Autodesk Fusion 360 part; units mm, degrees
sketch "Sketch1" plane through (0, 0, 0) normal (0, 0, 1) x (1, 0, 0)
  line L0 (0, 0) -> (70, 0)
  line L1 (70, 0) -> (70, 70)
  line L2 (70, 70) -> (0, 70)
  line L3 (0, 70) -> (0, 0)
  circle A0 centre (7.5, 62.5) radius 1.75
  circle A1 centre (62.5, 62.5) radius 1.75
  circle A2 centre (7.5, 7.5) radius 1.75
  circle A3 centre (62.5, 7.5) radius 1.75
  dimension "d1" = 70
  dimension "d2" = 70
  dimension "d3" = 3.5
  dimension "d4" = 7.5
  dimension "d5" = 7.5
  dimension "d8" = 55
  dimension "d9" = -55
extrude "Extrude1" add sketch "Sketch1" along normal blind 5
sketch "Sketch2" plane through (0, 0, 5) normal (0, 0, 1) x (-1, 0, 0)
  circle A0 centre (-62.5, -7.5) radius 1.75
  circle A1 centre (-7.5, -62.5) radius 1.75
  circle A2 centre (-7.5, -7.5) radius 1.75
  circle A3 centre (-62.5, -62.5) radius 1.75
  line L0 (0, -70) -> (0, 0)
  line L1 (0, 0) -> (-70, 0)
  line L2 (-70, 0) -> (-70, -70)
  line L3 (-70, -70) -> (0, -70)
  circle A4 centre (-35, -35) radius 11.4
  dimension "d12" = 22.8
extrude "Extrude2" cut sketch "Sketch2" against normal blind 5 contours A4
sketch "Sketch3" plane through (0, 0, 5) normal (0, 0, 1) x (-1, 0, 0)
  circle A0 centre (-35, -35) radius 11.4
  circle A1 centre (-62.5, -7.5) radius 1.75
  circle A2 centre (-7.5, -62.5) radius 1.75
  circle A3 centre (-7.5, -7.5) radius 1.75
  circle A4 centre (-62.5, -62.5) radius 1.75
  line L0 (0, -70) -> (0, 0)
  line L1 (0, 0) -> (-70, 0)
  line L2 (-70, 0) -> (-70, -70)
  line L3 (-70, -70) -> (0, -70)
  circle A5 centre (-35, -35) radius 16
  dimension "d15" = 32
extrude "Extrude3" add sketch "Sketch3" along normal blind 15 contours A0 | A5
sketch "Sketch4" plane through (0, 0, 20) normal (0, 0, 1) x (-1, 0, 0)
  circle A0 centre (-35, -35) radius 16
  circle A1 centre (-35, -35) radius 4.5
  dimension "d18" = 9
extrude "Extrude4" cut sketch "Sketch4" against normal blind 45 contours A1
sketch "Sketch5" plane through (0, 0, 20) normal (0, 0, 1) x (-1, 0, 0)
  circle A0 centre (-35, -35) radius 4.5
  circle A1 centre (-35, -35) radius 16
  circle A2 centre (-35, -35) radius 11.4
  dimension "d21" = 22.8
extrude "Extrude5" cut sketch "Sketch5" against normal blind 6 contours A2
extrude "Extrude6" add 1 faces at (25.9592, 35.7899, 5) along direction (0, 0, -1) blind 3.5
chamfer "Chamfer1" distance 6 angle 45 2 edges at (39.1955, 36.6273, 14) (39.1955, 36.6273, 1.5)
fillet "Fillet2" radius 65 1 edges at (0, 0, 2.5)
fillet "Fillet3" radius 5 3 edges at (70, 0, 2.5) (70, 70, 2.5) (0, 70, 2.5)
Here's how the part is built. I have some questions about the finished solid (model axes, mm). A direction names the side the tool comes from. Round coordinates to 2 decimals unless told otherwise and drop trailing zeros. Write each loop counter-clockwise with the first axis right and the second up, starting at its lowest first coordinate (ties: lowest second). Pieces come first, ordered by that corner, then holes.
1. Suppose I cut it at A-A (x = 35). List the corners of the cut face in (y, z) for me, and give its area (3 significant figures).
2. For faces 1 (the cylindrical face through (7.12, 64.21, 2.46)), 2 (the cylindrical face through (46.39, 34.5, 17.04)), 3 (the cylindrical face through (46.39, 34.5, 0.76)), which set-ups out of +Z, -Z, +X, -X, +Y, -Y let a thin tool reach every point of the face, with its end or its side?
3. Suppose I cut it at C-C (z = 2.75). State how many separate pieces and enclosed holes the cut face has, and give its area (3 significant figures).
4. If we mould it in two halves opening along Y, with no side actions, what happens to faces 4 (the cylindrical face through (50.985, 35.703, 12.395)), 5 (the cylindrical face through (64.169, 6.974, 2.465)), 6 (the flat face through (50, 43, 0)), 7 (the conical face through (40, 35, 7))? For each: released by +Y, released by -Y, zero draft, split by the parting line, or undercut.
5. Will these pins go through, and if not, where does the flat tip stop? pin 1 Ø1.5 at (y, z) = (61, 3) entering from -X; pin 2 Ø4 at (x, y) = (15.5, 27.5) entering from +Z; pin 3 Ø11.5 at (x, y) = (36, 31) entering from +Z.
6. I need wall thicknesses on L1, parallel to Y at x = 35, z = 7.8; L2, parallel to X at y = 35, z = 17.85; L3, parallel to Z at x = 50.5, y = 20.5. Which ranges of each line are inside material? Lowest first, please.
7. Suppose I cut it at B-B (y = 62.5). List the corners of the cut face in (x, z) for me.
Answer sheet:
1. outline: (7.34, 0) - (23.6, 0) - (23.6, 1.5) - (24.5, 1.5) - (30.5, 7.5) - (30.5, 8) - (24.5, 14) - (23.6, 14) - (23.6, 20) - (19, 20) - (19, 5) - (7.34, 5) - close; (39.5, 7.5) - (45.5, 1.5) - (46.4, 1.5) - (46.4, 0) - (70, 0) - (70, 5) - (51, 5) - (51, 20) - (46.4, 20) - (46.4, 14) - (45.5, 14) - (39.5, 8) - close
1. area: 438 mm2
2. face 1: +Z, -Z
2. face 2: +Z
2. face 3: -Z
3. separate pieces: 1
3. enclosed holes: 4
3. area: 3,680 mm2
4. face 4: split by the parting line
4. face 5: undercut
4. face 6: zero draft
4. face 7: undercut
5. pin 1: stops at x = 0.08
5. pin 2: stops at z = 5
5. pin 3: stops at z = 13.37
6. L1: y = 19 to 30.5, 39.5 to 51
6. L2: x = 19 to 23.6, 46.4 to 51
6. L3: z = 0 to 5
7. outline: (0.05, 0) - (5.75, 0) - (5.75, 5) - (0.05, 5) - close; (9.25, 0) - (60.75, 0) - (60.75, 5) - (9.25, 5) - close; (64.25, 0) - (70, 0) - (70, 5) - (64.25, 5) - close
